from build123d import *

# Parameters (mm, degrees)
F1_DEPTH = 1.5875


# Not quite as in the source:
# - a feature names something its author has since deleted; it is built from what else it names


with BuildPart() as f1:
    # F0 (on Right) → F1 (new body)
    with BuildSketch(Plane.YZ):
        with BuildLine():
            ThreePointArc((-22.32025, 0.0538603849), (-22.5590646592, -0.5136656763), (-23.1318048474, -0.739689897))
            Line((-23.1318048474, -0.739689897), (24.5522451458, -9.5030463267))
            Line((24.5522451458, -9.5030463267), (23.9059205272, 0))
            ThreePointArc((23.9059205272, 0), (23.9072925, -0.0269146615), (23.90775, -0.0538603849))
            ThreePointArc((23.90775, -0.0538603849), (23.0870542766, -0.8471528848), (22.3220794728, 0))
            Line((22.3220794728, 0), (21.7877844548, -7.8558516301))
            Line((21.7877844548, -7.8558516301), (-22.8339183638, 0.796553686))
            ThreePointArc((-22.8339183638, 0.796553686), (-22.461177719, 0.5053713282), (-22.32025, 0.0538603849))
        make_face()
        with BuildLine():
            Line((-23.0961951526, 0.8474106668), (-23.1318048474, -0.739689897))
            ThreePointArc((-23.1318048474, -0.739689897), (-22.5590646592, -0.5136656763), (-22.32025, 0.0538603849))
            ThreePointArc((-22.32025, 0.0538603849), (-22.461177719, 0.5053713282), (-22.8339183638, 0.796553686))
            Line((-22.8339183638, 0.796553686), (-23.0961951526, 0.8474106668))
        make_face()
        with BuildLine():
            ThreePointArc((-23.0961951526, 0.8474106668), (-23.9075502819, 0.0716652323), (-23.1318048474, -0.739689897))
            Line((-23.1318048474, -0.739689897), (-23.0961951526, 0.8474106668))
        make_face()
    extrude(amount=F1_DEPTH)


solid = f1.part
Can you work these out from the model? Positions are in its coordinate system, mm. A direction names the side the tool comes from. Coordinates: 2 decimals unless noted, no trailing zeros. Order: outer loops, then holes, each group sorted by start corner. A loop starts at its lowest first (then second) coordinate and runs counter-clockwise, first axis right, second up. Notation, with made-up numbers: (-18, 53.25) - (17, 53.25) arc R28 cw to (17, 91.25) - close; hole circle Ø9 at (4.5, 24.5). An arc over 180 degrees is marked (long way). Answer as a JSON object with one key per item and string values. Group by question number.
Q1. Imagine slicing it at A-A (z = -7.25). Please give me the cut outline in (x, y), and give its area (3 significant figures).
Q2. Imagine slicing it at C-C (z = -2.5). Please give me the cut outline in (x, y), and give its area (3 significant figures).
Q3. I need wall thicknesses on line 1 (Z direction, x = 0.1, y = -1); line 2 (Z direction, x = 0.1, y = 15). Which ranges of each line are inside material? Lowest first, please. Write a range as from..to.
Q4. On a 3-axis mill with a long thin cutter (end or side, diameter ignored), from which of +Z, -Z, +X, -X, +Y, -Y can I reach the whole of each face in a straight line? I mean faces 1 (the face through (0.78, 22.06, -3.87)), 2 (the face through (0, 2, -4.3)). Say none if no direction works.
Q5. Imagine slicing it at D-D (y = -11). Please give me the cut outline in (x, z).
Q6. Imagine slicing it at B-B (x = 0.3). Please give me the cut outline in (y, z), and give its area (3 significant figures).
Determined:
{
 "1": {"outline": "(0, 12.29) - (1.59, 12.29) - (1.59, 18.66) - (0, 18.66) - close; (0, 21.83) - (1.59, 21.83) - (1.59, 24.4) - (0, 24.4) - close", "area": "14.2 mm2"},
 "2": {"outline": "(0, -13.55) - (1.59, -13.55) - (1.59, -5.83) - (0, -5.83) - close; (0, 22.15) - (1.59, 22.15) - (1.59, 24.08) - (0, 24.08) - close", "area": "15.3 mm2"},
 "3": {"line 1": "z = -4.81..-3.44", "line 2": "z = -7.75..-6.54"},
 "4": {"face 1": "+Z, +X, -X", "face 2": "+Z, -Z, -X, +Y, -Y"},
 "5": {"outline": "(0, -2.97) - (1.59, -2.97) - (1.59, -1.5) - (0, -1.5) - close"},
 "6": {"outline": "(-23.13, -0.74) - (24.55, -9.5) - (23.91, 0) arc R0.79 cw (long way) to (22.32, 0) - (21.79, -7.86) - (-23.1, 0.85) arc R0.79 ccw to start", "area": "81.7 mm2"}
}
